Can you work these out from the model? Positions are in its coordinate system, mm. Give positions to 0.01 mm unless a question says otherwise; leave off trailing zeros.
Autodesk Inventor part; units mm, degrees
ref_plane "YZ Plane" through (0, 0, 0) normal (1, 0, 0) x (0, 1, 0)
ref_plane "XZ Plane" through (0, 0, 0) normal (0, 1, 0) x (-1, 0, 0)
ref_plane "XY Plane" through (0, 0, 0) normal (0, 0, 1) x (1, 0, 0)
sketch "스케치1" plane through (0, 0, 0) normal (0, 0, 1) x (1, 0, 0)
  line L0 (-9.7, -10) -> (9.7, -10)
  line L1 (10, -9.7) -> (10, 9.7)
  line L2 (9.7, 10) -> (-9.7, 10)
  line L3 (-10, 9.7) -> (-10, -9.7)
  line L4 (-10, -10) -> (10, 10) construction
  line L5 (10, -10) -> (-10, 10) construction
  circle A0 centre (-7, 7) radius 2
  line L6 (0, 15.6683) -> (0, -20)
  line L7 (-22.0072, 0) -> (22.0072, 0)
  circle A1 centre (0, 0) radius 2.15
  arc A2 (-9.7, 10) -> (-10, 9.7) centre (-9.7, 9.7) ccw
  arc A3 (10, 9.7) -> (9.7, 10) centre (9.7, 9.7) ccw
  arc A4 (9.7, -10) -> (10, -9.7) centre (9.7, -9.7) ccw
  arc A5 (-10, -9.7) -> (-9.7, -10) centre (-9.7, -9.7) ccw
  line L8 (-2.65, 10) -> (-2.65, 8.5)
  line L9 (-2.65, 8.5) -> (-4.15, 8.5)
  line L10 (-4.15, 8.5) -> (-4.15, 4.8)
  line L11 (4.15, 4.8) -> (4.15, 8.5)
  line L12 (4.15, 8.5) -> (2.65, 8.5)
  line L13 (2.65, 8.5) -> (2.65, 10)
  line L14 (-0.1, 3.3008) -> (0, 3.2)
  line L15 (0.1, 3.3008) -> (0, 3.2)
  arc A6 (-4.15, 4.8) -> (-0.1, 3.3008) centre (0, 9.7908) ccw
  arc A7 (0.1, 3.3008) -> (4.15, 4.8) centre (0, 9.7908) ccw
  circle A8 centre (7, 7) radius 2
  circle A9 centre (-7, -7) radius 2
  circle A10 centre (7, -7) radius 2
  line L16 (-3.3008, 0.1) -> (-3.2, 0)
  line L17 (-3.3008, -0.1) -> (-3.2, 0)
  arc A11 (-4.8, -4.15) -> (-3.3008, -0.1) centre (-9.7908, 0) ccw
  line L18 (-8.5, -4.15) -> (-4.8, -4.15)
  line L19 (-10, -2.65) -> (-8.5, -2.65)
  line L20 (-8.5, 2.65) -> (-10, 2.65)
  arc A12 (-3.3008, 0.1) -> (-4.8, 4.15) centre (-9.7908, 0) ccw
  line L21 (-4.8, 4.15) -> (-8.5, 4.15)
  line L22 (-8.5, 4.15) -> (-8.5, 2.65)
  line L23 (-8.5, -2.65) -> (-8.5, -4.15)
  line L24 (-0.1, -3.3008) -> (0, -3.2)
  line L25 (0.1, -3.3008) -> (0, -3.2)
  arc A13 (4.15, -4.8) -> (0.1, -3.3008) centre (0, -9.7908) ccw
  line L26 (4.15, -8.5) -> (4.15, -4.8)
  line L27 (2.65, -10) -> (2.65, -8.5)
  line L28 (-2.65, -8.5) -> (-2.65, -10)
  arc A14 (-0.1, -3.3008) -> (-4.15, -4.8) centre (0, -9.7908) ccw
  line L29 (-4.15, -4.8) -> (-4.15, -8.5)
  line L30 (-4.15, -8.5) -> (-2.65, -8.5)
  line L31 (2.65, -8.5) -> (4.15, -8.5)
  line L32 (3.3008, -0.1) -> (3.2, 0)
  line L33 (3.3008, 0.1) -> (3.2, 0)
  arc A15 (4.8, 4.15) -> (3.3008, 0.1) centre (9.7908, 0) ccw
  line L34 (8.5, 4.15) -> (4.8, 4.15)
  line L35 (10, 2.65) -> (8.5, 2.65)
  line L36 (8.5, -2.65) -> (10, -2.65)
  arc A16 (3.3008, -0.1) -> (4.8, -4.15) centre (9.7908, 0) ccw
  line L37 (4.8, -4.15) -> (8.5, -4.15)
  line L38 (8.5, -4.15) -> (8.5, -2.65)
  line L39 (8.5, 2.65) -> (8.5, 4.15)
  point P0 (2.65, 9.25)
  point P1 (-2.65, 9.25)
  point P2 (-4.15, 6.65)
  point P3 (0, 3.3)
  point P4 (-3.3, 0)
  point P5 (-9.25, -2.65)
  point P6 (-6.65, -4.15)
  point P7 (-9.25, 2.65)
  point P8 (0, -3.3)
  point P9 (2.65, -9.25)
  point P10 (4.15, -6.65)
  point P11 (-2.65, -9.25)
  point P12 (3.3, 0)
  point P13 (9.25, 2.65)
  point P14 (6.65, 4.15)
  point P15 (9.25, -2.65)
  dimension "d0" = 20
  dimension "d1" = 20
  dimension "d2" = 4
  dimension "d3" = 14
  dimension "d4" = 14
  dimension "d5" = 4.3
  dimension "d6" = 0.3
  dimension "d9" = 8.3
  dimension "d10" = 5.3
  dimension "d11" = 5.3
  dimension "d12" = 1.5
  dimension "d15" = 0.1
  dimension "d16" = 0.1
  dimension "d17" = 0.1
  dimension "d19" = 3.7
  dimension "d22" = 360
extrude "프로파일 길이 설정" add sketch "스케치1" along normal blind 550 contours A5 L3 L19 L23 L18 A11 L17 L7 A1 L6 L24 A14 L29 L30 L28 L0 | L27 L31 L26 A13 L25 L6 A1 L7 L32 A16 L37 L38 L36 L1 A4 L0 | L3 A2 L2 L8 L9 L10 A6 L14 L6 A1 L7 L16 A12 L21 L22 L20 | A1 L6 L15 A7 L11 L12 L13 L2 A3 L1 L35 L39 L34 A15 L33 L7
fillet "모서리" radius 0.05 32 edges at (10, 2.65, 275) (8.5, 2.65, 275) (8.5, 4.15, 275) (10, -2.65, 275) (8.5, -2.65, 275) (8.5, -4.15, 275) (2.65, 8.5, 275) (2.65, 10, 275) (4.15, 8.5, 275) (-4.15, 8.5, 275) (-2.65, 8.5, 275) (-2.65, 10, 275) (-10, 2.65, 275) (-8.5, 2.65, 275) (-8.5, 4.15, 275) (-8.5, -4.15, 275) (-8.5, -2.65, 275) (-10, -2.65, 275) (-2.65, -10, 275) (-2.65, -8.5, 275) (-4.15, -8.5, 275) (2.65, -8.5, 275) (4.15, -8.5, 275) (2.65, -10, 275) (4.15, -4.8, 275) (-4.15, -4.8, 275) (-4.8, -4.15, 275) (-4.8, 4.15, 275) (-4.15, 4.8, 275) (4.15, 4.8, 275) (4.8, -4.15, 275) (4.8, 4.15, 275)
equation "\"d0\" = d1"
equation "\"d11\" = d10"
properties part number "20x20x550"
(1) If I drill on L1, parallel to Y at x = 7, z = 229.5; L2, parallel to Y at x = 3, z = 420.5; L3, parallel to Y at x = -6.5, z = 124, over which ranges is the centre line in solid material (lowest first)?
Returned:
L1: y = -10 to -9, -5 to -4.15, 4.15 to 5, 9 to 10
L2: y = -10 to -8.5, -4.03 to 4.03, 8.5 to 10
L3: y = -10 to -8.94, -5.06 to -4.15, 4.15 to 5.06, 8.94 to 10
(2) Will this pin go through, and if not, where does the flat tip stop? P1, Ø1.5, axis at x = 7.5, y = -7, coming from the -Z side.
Returned:
P1: passes through
(3) Imagine slicing it at A-A, the plane z = 516. Give the number of separate pieces and of enclosed holes in the cut face, plus the area to 3 significant figures.
Returned:
separate pieces: 1
enclosed holes: 5
area: 146 mm2
